Can you work these out from the model? Positions are in its coordinate system, mm. Give positions to 0.01 mm unless a question says otherwise; leave off trailing zeros. Loops run counter-clockwise (first coordinate to the right, second up) from the corner with the lowest first, then second, coordinate; pieces in that order, holes last. Notation, with made-up numbers: (-10.5, 50) - (16.5, 50) arc R23 ccw to (16.5, 82) - close; hole circle Ø3 at (33.5, 79.25). An arc over 180 degrees is marked (long way). Write item = value, one per line.
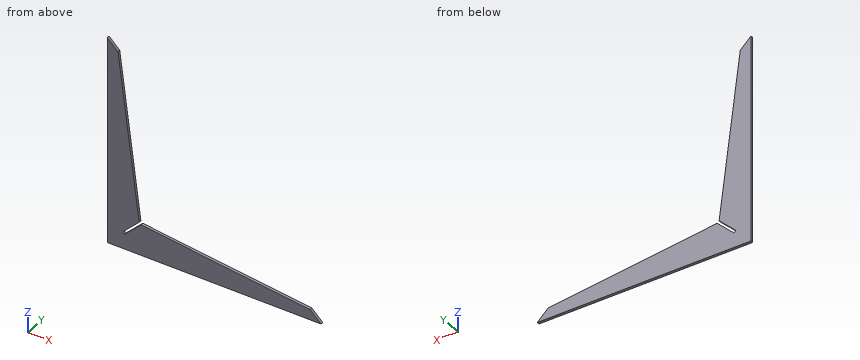
from build123d import *

# Parameters (mm, degrees)
F1_DEPTH = 12.7
F3_DEPTH = 25.4


# Not quite as in the source:
# - a length typed as a fraction of an inch, garbled in the dataset ("3 / 203.2 mm" for 3/8 in), is restored


with BuildPart() as f1:
    # F0 (on Front) → F1 (new body)
    with BuildSketch(Plane.XZ):
        Polygon((-313.2666666667, 601.1333333333), (-364.0666666667, 651.9333333333), (-364.0666666667, -364.0666666667), (651.9333333333, -364.0666666667), (601.1333333333, -313.2666666667), (-211.6666666667, -211.6666666667), align=None)
    extrude(amount=F1_DEPTH)

    # F2 (on face) → F3 (cut)
    with BuildSketch(Plane.XZ.offset(12.7)):
        Polygon((-292.3567947272, -283.3765386061), (-287.8666666667, -287.8666666667), (-283.3765386061, -292.3567947272), (-203.6842167813, -212.6644729023), (-212.6644729023, -203.6842167813), align=None)
    extrude(amount=-F3_DEPTH, mode=Mode.SUBTRACT)


solid = f1.part
Q1. Imagine slicing it at B-B, the plane x = -253. Write out the boundary of the cut face in (y, z), then the cut area to 3 significant figures.
Output:
outline = (-12.7, -364.07) - (0, -364.07) - (0, -261.98) - (-12.7, -261.98) - close; (-12.7, -244.02) - (0, -244.02) - (0, 119) - (-12.7, 119) - close
area = 5,910 mm2
Q2. Imagine slicing it at A-A, the plane y = -10.5. Write out the boundary of the cut face in (x, z).
Output:
outline = (-364.07, -364.07) - (651.93, -364.07) - (601.13, -313.27) - (-203.68, -212.66) - (-283.38, -292.36) - (-292.36, -283.38) - (-212.66, -203.68) - (-313.27, 601.13) - (-364.07, 651.93) - close
Q3. For pin 1 (2 mm diameter, centred on y = -1.5, z = 274.5, fed in from +X); pin 2 (1.5 mm diameter, centred on x = 492.5, y = -5.5, fed in from +Z), each with a flat end and sliding along its axis, tell me the tip position at first contact or that it passes through.
Output:
pin_1 = -272.31
pin_2 = -299.59
Q4. Imagine slicing it at C-C, the plane z = 217. Write out the boundary of the cut face in (x, y), then the cut area to 3 significant figures.
Output:
outline = (-364.07, -12.7) - (-265.25, -12.7) - (-265.25, 0) - (-364.07, 0) - close
area = 1,250 mm2
Q5. Imagine slicing it at D-D, the plane x = 367. Write out the boundary of the cut face in (y, z).
Output:
outline = (-12.7, -364.07) - (0, -364.07) - (0, -284) - (-12.7, -284) - close
Q6. I need wall thicknesses on L1, parallel to X at y = -10.5, z = -202 (3 decimals); L2, parallel to Z at x = -176.5, y = -7.25; L3, parallel to X at y = -1.5, z = 348 (3 decimals). Which ranges of each line are inside material? Lowest first, please.
Output:
L1 = -364.067 to -212.875
L2 = -364.07 to -216.06
L3 = -364.067 to -281.625
